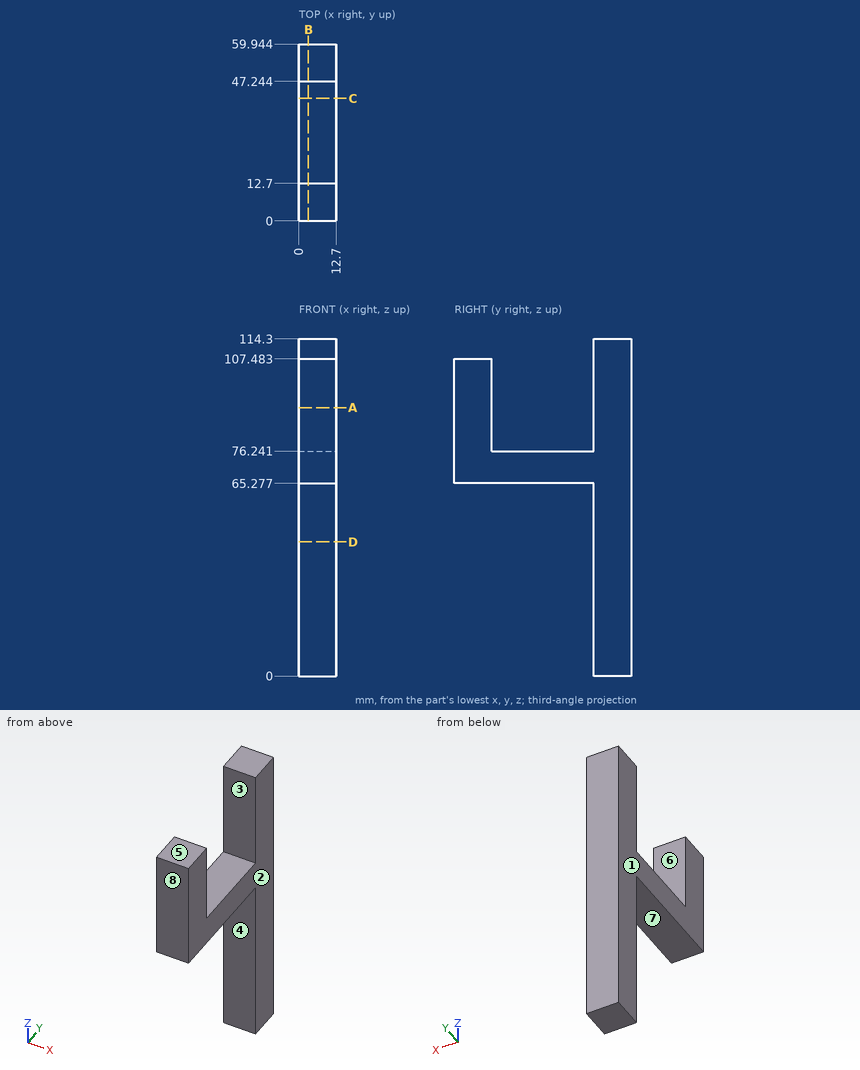
Geometry: see drawing. Coordinates: mm, zero at the bounding-box minimum. A direction names the side the tool comes from. Give positions to 0.01 mm unless a question says otherwise; leave off trailing zeros. Write each loop counter-clockwise with the first axis right and the second up, starting at its lowest first coordinate (ties: lowest second). Pieces come first, ordered by that corner, then holes. Notation, with made-up numbers: M 40.25,-21.75 L 55.25,-21.75 A11 ccw 55.25,-4.75 Z; hole C 73.5,4 d1. An arc over 180 degrees is marked long. Return JSON: item names as keys, results as strings. Group by question number.
1) Ray query, L1, parallel to Y at x = 4.25, z = 107; L2, parallel to Z at x = 2, y = 42; L3, parallel to Y at x = 5.25, z = 49. Return the intervals inside material, ascending.
2) First-contact query: pin 1 Ø3 at (y, z) = (44.5, 19.5) entering from +X; pin 2 Ø6.5 at (x, y) = (8, 22.5) entering from -Z. Flat tips, straight axial feed; report the tip coordinate or a pass-through.
3) Cut plane B-B, the plane x = 3.25. Output: boundary loops of the cut face in (y, z), then the cut area to 3 significant figures.
4) Cut plane C-C, the plane y = 41.5. Output: boundary loops of the cut face in (x, z).
5) Draft query along Y for the marked faces 6, 7 and 8. Return one class per face: released by +Y, released by -Y, zero draft, split by the parting line, or undercut.
6) Cut plane D-D, the plane z = 45.5. Output: boundary loops of the cut face in (x, y).
7) Cut plane A-A, the plane z = 91. Output: boundary loops of the cut face in (x, y).
8) Set-up query: the marked faces 1, 2, 3, 4 and 5. Return all of +Z, -Z, +X, -X, +Y, -Y with unobstructed straight access to the full face (end or side cutting, diameter ignored); none if empty.
Data:
{
 "1": {"L1": "y = 0 to 12.7, 47.24 to 59.94", "L2": "z = 65.28 to 76.24", "L3": "y = 47.24 to 59.94"},
 "2": {"pin 1": "passes through", "pin 2": "stops at z = 65.28"},
 "3": {"outline": "M 0,65.28 L 47.24,65.28 L 47.24,0 L 59.94,0 L 59.94,114.3 L 47.24,114.3 L 47.24,76.24 L 12.7,76.24 L 12.7,107.48 L 0,107.48 Z", "area": "2,370 mm²"},
 "4": {"outline": "M 0,65.28 L 12.7,65.28 L 12.7,76.24 L 0,76.24 Z"},
 "5": {"face 6": "undercut", "face 7": "zero draft", "face 8": "released by -Y"},
 "6": {"outline": "M 0,47.24 L 12.7,47.24 L 12.7,59.94 L 0,59.94 Z"},
 "7": {"outline": "M 0,0 L 12.7,0 L 12.7,12.7 L 0,12.7 Z; M 0,47.24 L 12.7,47.24 L 12.7,59.94 L 0,59.94 Z"},
 "8": {"face 1": "+Z, -Z, -X, +Y, -Y", "face 2": "+Z, -Z, +X, +Y, -Y", "face 3": "+Z, +X, -X", "face 4": "-Z, +X, -X, -Y", "face 5": "+Z, +X, -X, -Y"}
}
